Design review of the part built by this model. Coordinates are the model's own, in mm. Face numbers are marked on the shaded views. A direction names the side the tool comes from. Round coordinates to 2 decimals unless told otherwise and drop trailing zeros. Order: outer loops, then holes, each group sorted by start corner. A loop starts at its lowest first (then second) coordinate and runs counter-clockwise, first axis right, second up.
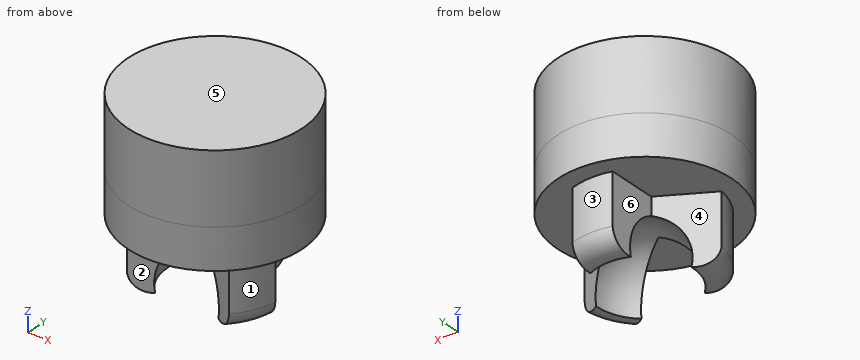
from build123d import *

# Parameters (mm, degrees)
CORTE_EXTRUS_O1_DEPTH    = 12.838758968
ESBO_O4_R                = 1.6
RESSALTO_EXTRUS_O1_DEPTH = 4
ESBO_O5_W                = 57.361933027
ESBO_O5_H                = 29.217059345
ESBO_O5_R                = 10
CORTE_EXTRUS_O2_DEPTH    = 10
ESBO_O6_R                = 10
ESBO_O6_R_2              = 8.625
CORTE_EXTRUS_O3_DEPTH    = 10
ESBO_O8_R                = 8.625
RESSALTO_EXTRUS_O2_DEPTH = 7


with BuildPart() as part:
    # Esboço1 → Revolução1 (revolve)
    with BuildSketch(Plane(origin=(0, 0, 0), x_dir=(1, 0, 0), z_dir=(0, 1, 0))):
        with BuildLine():
            Line((0, 0), (6.891534421, 0))
            Line((6.891534421, 0), (6.891534421, 5))
            ThreePointArc((6.891534421, 5), (6.180613943, 6.309516298), (4.743586175, 6.703460527))
            ThreePointArc((4.743586175, 6.703460527), (3.710745118, 2.736851933), (0, 0.995842151))
            Line((0, 0.995842151), (0, 0))
        make_face()
    revolve(axis=Axis((0, 0, 0), (0, 0, -1)))

    # Esboço3 → Corte-extrusão1 (cut, through all)
    with BuildSketch(Plane.XY):
        with BuildLine():
            Line((-2, 19.326317369), (-2, 1.734101615))
            Line((-2, 1.734101615), (-17.937282026, -7.467292453))
            ThreePointArc((-17.937282026, -7.467292453), (-16.698748021, 9.932691356), (-2, 19.326317369))
        make_face()
        with BuildLine():
            Line((2, 19.326317369), (2, 1.734101615))
            Line((2, 1.734101615), (17.937282026, -7.467292453))
            ThreePointArc((17.937282026, -7.467292453), (16.698748021, 9.932691356), (2, 19.326317369))
        make_face()
        with BuildLine():
            Line((0, -1.73), (-16.027252382, -10.983338477))
            ThreePointArc((-16.027252382, -10.983338477), (0, -19.429527607), (16.027252382, -10.983338477))
            Line((16.027252382, -10.983338477), (0, -1.73))
        make_face()
    extrude(amount=-CORTE_EXTRUS_O1_DEPTH, mode=Mode.SUBTRACT)

    # Esboço4 → Ressalto-extrusão1 (add)
    with BuildSketch(Plane.XY):
        with BuildLine():
            ThreePointArc((-6.64, -7.477325725), (0, -10), (6.64, -7.477325725))
            ThreePointArc((6.64, -7.477325725), (12.553949294, -4.249302623), (19.284210526, -3.935434592))
            ThreePointArc((19.284210526, -3.935434592), (24, 0), (19.284210526, 3.935434592))
            ThreePointArc((19.284210526, 3.935434592), (12.553949294, 4.249302623), (6.64, 7.477325725))
            ThreePointArc((6.64, 7.477325725), (0, 10), (-6.64, 7.477325725))
            ThreePointArc((-6.64, 7.477325725), (-12.553949294, 4.249302623), (-19.284210526, 3.935434592))
            ThreePointArc((-19.284210526, 3.935434592), (-24, 0), (-19.284210526, -3.935434592))
            ThreePointArc((-19.284210526, -3.935434592), (-12.553949294, -4.249302623), (-6.64, -7.477325725))
        make_face()
        with Locations((20, 0)):
            Circle(ESBO_O4_R, mode=Mode.SUBTRACT)
        with Locations((-20, 0)):
            Circle(ESBO_O4_R, mode=Mode.SUBTRACT)
    extrude(amount=RESSALTO_EXTRUS_O1_DEPTH)

    # Esboço5 → Corte-extrusão2 (cut)
    with BuildSketch(Plane(origin=(0, 0, 0), x_dir=(-1, 0, 0), z_dir=(0, 0, -1))):
        with Locations((1.250708993, 0.03640394)):
            Rectangle(ESBO_O5_W, ESBO_O5_H)
        with Locations(Location((0, 0, 0), (0, 0, 180))):
            Circle(ESBO_O5_R, mode=Mode.SUBTRACT)
    extrude(amount=-CORTE_EXTRUS_O2_DEPTH, mode=Mode.SUBTRACT)

    # Esboço6 → Corte-extrusão3 (cut)
    with BuildSketch(Plane(origin=(0, 0, 0), x_dir=(-1, 0, 0), z_dir=(0, 0, -1))):
        Circle(ESBO_O6_R)
        Circle(ESBO_O6_R_2, mode=Mode.SUBTRACT)
    extrude(amount=-CORTE_EXTRUS_O3_DEPTH, mode=Mode.SUBTRACT)

    # Esboço8 → Ressalto-extrusão2 (add)
    with BuildSketch(Plane.XY.offset(4)):
        with Locations(Location((0, 0, 0), (0, 0, 180))):
            Circle(ESBO_O8_R)
    extrude(amount=RESSALTO_EXTRUS_O2_DEPTH)


solid = part.part
1) Take a section at D-D on y = 3.25. Give the boundary of the cut face in (x, z), plus the area to 3 significant figures.
Results:
outline: (-7.99, 0) - (-2, 0) - (-2, -2.87) arc R3.57 cw to (2, -2.87) - (2, 0) - (7.99, 0) - (7.99, 11) - (-7.99, 11) - close
area: 186 mm2
2) Take a section at A-A on z = -2.25. Give the boundary of the cut face in (x, y).
Results:
outline: (-6.81, -1.04) arc R6.89 ccw to (-5.08, -4.66) - (-1.74, -2.74) arc R3.24 cw to (-3.04, 1.13) - close; (-2, 2.56) arc R3.24 cw to (2, 2.56) - (2, 6.59) arc R6.89 ccw to (-2, 6.59) - close; (1.74, -2.74) - (5.08, -4.66) arc R6.89 ccw to (6.81, -1.04) - (3.04, 1.13) arc R3.24 cw to start
3) The part is to be moulded in two halves that separate along X. For the marked faces 1, 2, 3 and 4, say which applies: released by +X, released by -X, zero draft, split by the parting line, or undercut.
Results:
face 1: released by +X
face 2: undercut
face 3: split by the parting line
face 4: released by -X
4) Clearance check with flat-ended pins moving along their axes: P1, Ø1, axis at x = 6, z = -4.5, coming from the -Y side; P2, Ø1, axis at x = 6.5, z = 7, coming from the -Y side; P3, Ø5.5, axis at y = 4.5, z = -4, coming from the +X side. State where each tip first meets the part, or that it passes through.
Results:
P1: stops at y = -4.15
P2: stops at y = -6.2
P3: stops at x = 2
5) To check wall thickness, follow line 1 along Z through (x, y) = (-7, -0.25); line 2 along X through (y, z) = (-4, -3); line 3 along Y through (x, z) = (0.25, 7.75). State the ranges of each line that lie inside material, in increasing order.
Results:
line 1: z = 0 to 11
line 2: x = -5.61 to -3.93, 3.93 to 5.61
line 3: y = -8.62 to 8.62
6) Take a section at C-C on z = 5.25. Give the boundary of the cut face in (x, y) (3 decimals), plus the area to 3 significant figures.
Results:
outline: circle Ø17.25 at (0, 0)
area: 234 mm2
7) For the marked faces 5 and 6, list the 3-axis set-ups (+Z, -Z, +X, -X, +Y, -Y) from which the entire face can be reached by the end or side of a thin tool; tool diameter is ignored.
Results:
face 5: +Z, +X, -X, +Y, -Y
face 6: -Z, -X, +Y
8) Take a section at B-B on y = 0.5. Give the boundary of the cut face in (x, z), plus the area to 3 significant figures.
Results:
outline: (-8.61, 0) - (-4.14, 0) - (-4.14, -3.39) arc R4.8 cw to (4.14, -3.39) - (4.14, 0) - (8.61, 0) - (8.61, 11) - (-8.61, 11) - close
area: 204 mm2
